Could you check a few things on this model? Use its own coordinates, in mm. Give positions to 0.01 mm unless a question says otherwise; leave off trailing zeros. Order: outer loops, then holes, each group sorted by start corner. A loop starts at its lowest first (then second) coordinate and runs counter-clockwise, first axis right, second up.
(1) Will these pins go through, and if not, where does the flat tip stop? pin 1 (2 mm diameter, centred on x = 35.5, z = -5.5, fed in from -Y); pin 2 (4 mm diameter, centred on x = 109.5, y = -6, fed in from +Z); pin 3 (1.5 mm diameter, centred on x = 64.5, y = 6, fed in from +Z).
(2) Imagine slicing it at A-A, the plane x = 76. Write out the boundary of the cut face in (y, z) (1 decimal).
(3) If I drill on probe 1 along Y at (x, z) = (96.5, 12.5); probe 2 along Y at (x, z) = (26, -6.5); probe 3 along X at (y, z) = (15.5, -6), over which ranges is the centre line in solid material (lowest first)?
Autodesk Inventor part; units mm, degrees
ref_plane "Start Plane" through (0, 0, 0) normal (1, 0, 0) x (0, 1, 0)
ref_plane "XZ Plane" through (0, 0, 0) normal (0, 1, 0) x (-1, 0, 0)
ref_plane "XY Plane" through (0, 0, 0) normal (0, 0, 1) x (1, 0, 0)
sketch "Main Sketch" plane through (0, 0, 0) normal (0, 0, 1) x (1, 0, 0)
  line L0 (0, 0) -> (132.08, 0)
  line L1 (0, 0) -> (0, 17.4625)
  line L2 (132.08, 17.4625) -> (132.08, 0)
  line L3 (0, 17.4625) -> (132.08, 17.4625)
  dimension "d3" = 34.925
revolve "Revolution1" add sketch "Main Sketch" angle 360 about axis through (0, 0, 0) along (1, 0, 0)
chamfer "Chamfer1" distance 2.54 angle 45 1 edges at (0, -17.4625, 0) measured on face at (88.0533, 17.4059, -1.4051)
fillet "Fillet1" radius 2.54 1 edges at (132.08, -17.4625, 0)
properties part number "Shaft" material "Steel"
Answer block:
1. pin 1: stops at y = -16.87
1. pin 2: stops at z = 17
1. pin 3: stops at z = 16.65
2. outline: circle Ø34.9 at (0, 0)
3. probe 1: y = -12.19 to 12.19
3. probe 2: y = -16.21 to 16.21
3. probe 3: x = 1.7 to 131.43
